Geometry check sheet. Reference: the model listing, model coordinates, mm. A direction names the side the tool comes from. Give positions to 0.01 mm unless a question says otherwise; leave off trailing zeros. Loops run counter-clockwise (first coordinate to the right, second up) from the corner with the lowest first, then second, coordinate; pieces in that order, holes last.
```python
from build123d import *

# Parameters (mm, degrees)
SKETCH1_R           = 82
BOSS_EXTRUDE1_DEPTH = 10
BOSS_EXTRUDE4_DEPTH = 220
BOSS_EXTRUDE5_START = -5
BOSS_EXTRUDE5_DEPTH = 5
SKETCH7_R           = 1
CUT_EXTRUDE1_DEPTH  = 12
CIRPATTERN1_COUNT   = 4


with BuildPart() as part:
    # Sketch1 → Boss-Extrude1 (new body)
    with BuildSketch(Plane(origin=(0, 0, 0), x_dir=(1, 0, 0), z_dir=(0, 1, 0))):
        with Locations(Location((0, 0, 0), (0, 0, 270))):
            Circle(SKETCH1_R)
    extrude(amount=BOSS_EXTRUDE1_DEPTH)

    # Sketch2 → Boss-Extrude4 (add)
    with BuildSketch(Plane(origin=(0, 10, 0), x_dir=(1, 0, 0), z_dir=(0, 1, 0))):
        with BuildLine():
            Line((-29.16066006, 62.535237306), (-31.273751369, 67.066776241))
            ThreePointArc((-31.273751369, 67.066776241), (0, 74), (31.273751369, 67.066776241))
            Line((31.273751369, 67.066776241), (29.16066006, 62.535237306))
            ThreePointArc((29.16066006, 62.535237306), (0, 69), (-29.16066006, 62.535237306))
        make_face()
    boss_extrude4 = extrude(amount=BOSS_EXTRUDE4_DEPTH)

    # Mirror2: Boss-Extrude4 across plane
    add(boss_extrude4.mirror(Plane.XY))

    # Sketch4 → Boss-Extrude5 (add)
    with BuildSketch(Plane(origin=(0, 230, 0), x_dir=(1, 0, 0), z_dir=(0, 1, 0)).offset(BOSS_EXTRUDE5_START)):
        with BuildLine():
            Line((-29.16066006, 62.535237306), (29.16066006, 62.535237306))
            ThreePointArc((29.16066006, 62.535237306), (0, 69), (-29.16066006, 62.535237306))
        make_face()
    boss_extrude5 = extrude(amount=BOSS_EXTRUDE5_DEPTH)

    # Mirror3: Boss-Extrude5 across plane
    add(boss_extrude5.mirror(Plane.XY))

    # Sketch7 → Cut-Extrude1 (cut)
    with BuildSketch(Plane(origin=(-57.982756057, 0, 57.982756057), x_dir=(0.7071067811865477, 0, 0.7071067811865475), z_dir=(-0.7071067811865475, 0, 0.7071067811865477))):
        with Locations((0, 5)):
            Circle(SKETCH7_R)
    cut_extrude1 = extrude(amount=-CUT_EXTRUDE1_DEPTH, mode=Mode.SUBTRACT)

    # CirPattern1: Cut-Extrude1 ×4 about axis
    cirpattern1_axis = Axis((0, 0, 0), (0, 1, 0))
    for i in range(1, CIRPATTERN1_COUNT):
        add(cut_extrude1.rotate(cirpattern1_axis, i * 360 / CIRPATTERN1_COUNT), mode=Mode.SUBTRACT)


solid = part.part
```
1) Sectioned sample at A-A on y = 43. Enter the section's corners in (x, z), plus the area to 3 significant figures.
2) Tool access check on faces 1 (the cylindrical face through (0, 116, -69)), 2 (the flat face through (0, 227, 62.535)), 3 (the flat face through (0, 230, 67)). Record the directions out of +Z, -Z, +X, -X, +Y, -Y that give a thin tool (end or side, any length) a straight path to the whole face; none if there is none.
3) Sectioned sample at C-C on z = 0. Enter the section's corners in (x, y).
4) Sectioned sample at D-D on z = 38. Enter the section's corners in (x, y).
5) Depth check by flat-ended pin: P1, Ø1.5, axis at x = 3.5, y = 228.5, coming from the +Z side; P2, Ø1.5, axis at x = 8.5, y = 227.5, coming from the -Z side; P3, Ø10, axis at x = -35.5, y = 101, coming from the -Z side. Enter the tip coordinate at first touch or a pass-through.
6) Sectioned sample at B-B on x = 0. Enter the section's corners in (y, z), plus the area to 3 significant figures.
7) Scan lines: line 1 along Y through (x, z) = (29, -21); line 2 along Z through (x, y) = (7.5, 38.5); line 3 along Z through (x, y) = (-27, 104.5). Record each from-to range of solid material in increasing order.
8) Mould release check, pull along Z, two halves, no side actions. Record for faces 4 (the cylindrical face through (0, 118, -74)), 5 (the cylindrical face through (0, 116, 69)), 6 (the cylindrical face through (0, 118, 74)), 7 (the flat face through (0, 225, 65)): +Z half, -Z half, draft (parallel to the pull), parting line (faces both ways), or undercut.
Determined:
1. outline: (-31.27, -67.07) arc R74 ccw to (31.27, -67.07) - (29.16, -62.54) arc R69 cw to (-29.16, -62.54) - close; (-31.27, 67.07) - (-29.16, 62.54) arc R69 cw to (29.16, 62.54) - (31.27, 67.07) arc R74 ccw to start
1. area: 624 mm2
2. face 1: none
2. face 2: +X, -X, +Y
2. face 3: +Z, -Z, +X, -X, +Y
3. outline: (-82, 0) - (82, 0) - (82, 10) - (-82, 10) - close
4. outline: (-72.66, 0) - (72.66, 0) - (72.66, 10) - (-72.66, 10) - close
5. P1: stops at z = 73.95
5. P2: stops at z = -73.59
5. P3: stops at z = -67.42
6. outline: (0, -82) - (10, -82) - (10, -74) - (230, -74) - (230, -62.54) - (225, -62.54) - (225, -69) - (10, -69) - (10, 69) - (225, 69) - (225, 62.54) - (230, 62.54) - (230, 74) - (10, 74) - (10, 82) - (0, 82) - close
6. area: 3,900 mm2
7. line 1: y = 0 to 10
7. line 2: z = -73.62 to -68.59, 68.59 to 73.62
7. line 3: z = -68.9 to -63.5, 63.5 to 68.9
8. face 4: -Z half
8. face 5: undercut
8. face 6: +Z half
8. face 7: undercut
